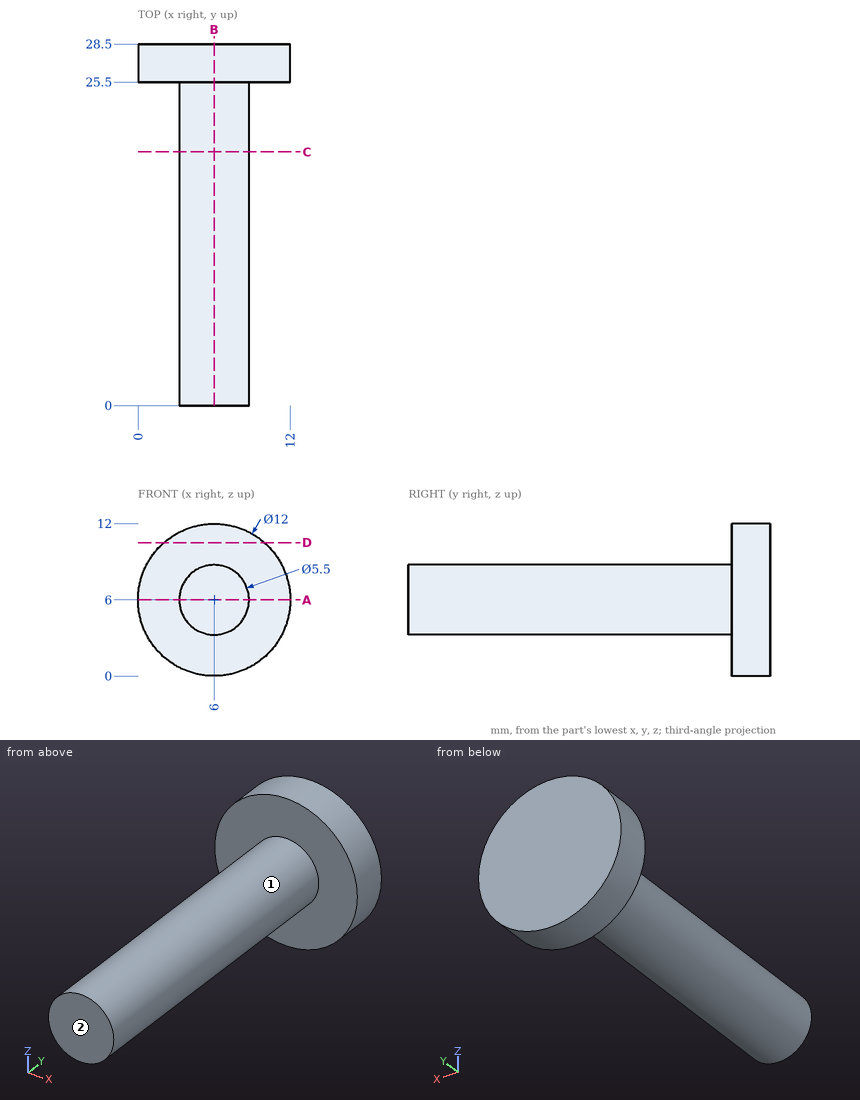
Source: three-view drawing plus pictorial views. Frame: mm from the lowest corner of the part. A direction names the side the tool comes from. Coordinates: 2 decimals unless noted, no trailing zeros. Write each loop counter-clockwise with the first axis right and the second up, starting at its lowest first coordinate (ties: lowest second). Pieces come first, ordered by that corner, then holes. Notation, with made-up numbers: (59.25, 29.5) -> (108.25, 29.5) arc R14 cw to (108.25, 42.5) -> close; hole circle Ø3 at (5.5, 49). An arc over 180 degrees is marked (long way). Answer as a JSON object with one key per item and string values.
1. First-contact query: P1, Ø2, axis at y = 25, z = 2.5, coming from the -X side; P2, Ø1.5, axis at x = 3.5, y = 24, coming from the -Z side. Flat tips, straight axial feed; report the tip coordinate or a pass-through.
Result set:
{"P1": "stops at x = 0.61", "P2": "stops at z = 3.88"}
2. Section C-C on y = 20. Return the cut outline in (x, z).
Result set:
{"outline": "circle Ø5.5 at (6, 6)"}
3. Section D-D on z = 10.5. Return the cut outline in (x, y).
Result set:
{"outline": "(2.03, 25.5) -> (9.97, 25.5) -> (9.97, 28.5) -> (2.03, 28.5) -> close"}
4. Section B-B on x = 6. Return the cut outline in (y, z).
Result set:
{"outline": "(0, 3.25) -> (25.5, 3.25) -> (25.5, 0) -> (28.5, 0) -> (28.5, 12) -> (25.5, 12) -> (25.5, 8.75) -> (0, 8.75) -> close"}
5. Section A-A on z = 6. Return the cut outline in (x, y).
Result set:
{"outline": "(0, 25.5) -> (3.25, 25.5) -> (3.25, 0) -> (8.75, 0) -> (8.75, 25.5) -> (12, 25.5) -> (12, 28.5) -> (0, 28.5) -> close"}
6. Access query for the marked faces 1 and 2. Directions: +Z, -Z, +X, -X, +Y, -Y. A direction counts if a zero-diameter tool reaches every point of the face in a straight line with its end or side. Return the directions, or none.
Result set:
{"face 1": "-Y", "face 2": "+Z, -Z, +X, -X, -Y"}
7. Material intervals for line 1 (Y direction, x = 10.5, z = 3.5); line 2 (Z direction, x = 7.25, y = 25.25); line 3 (Z direction, x = 7.75, y = 23.5), sorted ascending. Write a range as from..to.
Result set:
{"line 1": "y = 25.5..28.5", "line 2": "z = 3.55..8.45", "line 3": "z = 3.88..8.12"}
